```python
from build123d import *

# Parameters (mm, degrees)
EXTRUDE_1_DEPTH = 3.2
SKETCH_2_R      = 2.5
EXTRUDE_2_DEPTH = 25
CHAMFER_1_SIZE  = 1
CHAMFER_1_SIZE2 = 0.577350269


with BuildPart() as part:
    # Эскиз1 → Бобышка-Вытянуть1 (new body)
    with BuildSketch(Plane(origin=(0, 0, 0), x_dir=(1, 0, 0), z_dir=(0, 1, 0))):
        Polygon((4, -2.309401077), (4, 2.309401077), (0, 4.618802154), (-4, 2.309401077), (-4, -2.309401077), (0, -4.618802154), align=None)
    extrude(amount=EXTRUDE_1_DEPTH)

    # Эскиз2 → Бобышка-Вытянуть2 (add)
    with BuildSketch(Plane(origin=(0, 3.2, 0), x_dir=(1, 0, 0), z_dir=(0, 1, 0))):
        Circle(SKETCH_2_R)
    extrude(amount=EXTRUDE_2_DEPTH)

    # Фаска1
    chamfer_1_edges = [part.edges().sort_by_distance(p)[0] for p in [
        (-2, 0, 3.464101615),
        (-4, 0, 0),
        (-2, 0, -3.464101615),
        (2, 0, -3.464101615),
        (4, 0, 0),
        (2, 0, 3.464101615),
    ]]
    chamfer_1_side = [part.faces().sort_by_distance(p)[0] for p in [
        (0, 0, 0),
    ]]
    chamfer(chamfer_1_edges, length=CHAMFER_1_SIZE, length2=CHAMFER_1_SIZE2, reference=chamfer_1_side[0])


solid = part.part
```
The listing builds one solid part. Answer for the finished solid, in the listing's coordinates (mm). A direction names the side the tool comes from. Coordinates: 2 decimals unless noted, no trailing zeros. Write each loop counter-clockwise with the first axis right and the second up, starting at its lowest first coordinate (ties: lowest second). Pieces come first, ordered by that corner, then holes.
Q1. Section D-D, the plane z = 3 is taken. Write down the section's boundary in (x, y).
Returned:
outline: (-2.8, 0.58) - (-0.8, 0) - (0.8, 0) - (2.8, 0.58) - (2.8, 3.2) - (-2.8, 3.2) - close
Q2. Find the intervals of material crossed by line 1 along Y through (x, z) = (0, 2.75); line 2 along Y through (x, z) = (3.75, -0.5); line 3 along X through (y, z) = (4.75, 0), in increasing order.
Returned:
line 1: y = 0 to 3.2
line 2: y = 0.43 to 3.2
line 3: x = -2.5 to 2.5
Q3. Which of the six approach directions +Z, -Z, +X, -X, +Y, -Y give full straight-line access (tool end or side, diameter ignored) to faces 1 (the flat face through (2, 3.2, 2)), 2 (the flat face through (-1.725, 0.293, -3.053))?
Returned:
face 1: +Y
face 2: -Z, -X, -Y
Q4. Given P1, Ø1.5, axis at y = 19.5, z = 1.5, coming from the -X side; P2, Ø1, axis at x = -1, y = 8.5, coming from the +Z side; P3, Ø3, axis at y = 7.5, z = 3.5, coming from the -X side, each flat-ended and moving along its own axis, determine where each tip first touches the part or whether it passes through.
Returned:
P1: stops at x = -2.38
P2: stops at z = 2.45
P3: stops at x = -1.5
Q5. Section B-B, the plane x = 1.5 is taken. Write down the section's boundary in (y, z), then the cut area to 3 significant figures.
Returned:
outline: (0, -2.6) - (0.58, -3.75) - (3.2, -3.75) - (3.2, -2) - (28.2, -2) - (28.2, 2) - (3.2, 2) - (3.2, 3.75) - (0.58, 3.75) - (0, 2.6) - close
area: 123 mm2
Q6. Section C-C, the plane y = 19.25 is taken. Write down the section's boundary in (x, z).
Returned:
outline: circle Ø5 at (0, 0)
Q7. Section A-A, the plane z = 0 is taken. Write down the section's boundary in (x, y), then the cut area to 3 significant figures.
Returned:
outline: (-4, 0.58) - (-3, 0) - (3, 0) - (4, 0.58) - (4, 3.2) - (2.5, 3.2) - (2.5, 28.2) - (-2.5, 28.2) - (-2.5, 3.2) - (-4, 3.2) - close
area: 150 mm2
